from build123d import *

# Parameters (mm, degrees)
SKETCH_1_W             = 38
SKETCH_1_H             = 7
EXTRUDE_1_DEPTH        = 3
SKETCH_2_W             = 7
SKETCH_2_H             = 3
EXTRUDE_2_DEPTH        = 13
SKETCH_3_R             = 1.5
CUT_EXTRUDE_1_DEPTH    = 44.0464865
SKETCH_4_R             = 1.5
CUT_EXTRUDE_2_DEPTH    = 44.0464865
SKETCH_5_W             = 5
SKETCH_5_H             = 40.2
EXTRUDE_3_DEPTH        = 3
SKETCH_6_R             = 1.5
CUT_EXTRUDE_3_DEPTH    = 56.398916957
FILLET_1_R             = 5
FILLET_2_R             = 5
FILLET_2_OF_MIRROR_1_R = 5
SKETCH_7_W             = 73.096836427
SKETCH_7_H             = 5.118381576
CUT_EXTRUDE_4_DEPTH    = 13
SKETCH_9_W             = 54.2
SKETCH_9_H             = 3
EXTRUDE_4_DEPTH        = 1
SKETCH_8_R             = 1.5
CUT_EXTRUDE_5_DEPTH    = 61.669926652


with BuildPart() as part:
    # 草图1 → 凸台-拉伸1 (new body)
    with BuildSketch(Plane(origin=(0, 0, 0), x_dir=(1, 0, 0), z_dir=(0, 1, 0))):
        with Locations((-19, -3.5)):
            Rectangle(SKETCH_1_W, SKETCH_1_H)
    extrude_1 = extrude(amount=EXTRUDE_1_DEPTH)

    # 草图2 → 凸台-拉伸2 (add)
    with BuildSketch(Plane.XY.offset(7)):
        with Locations((-3.5, 1.5)):
            Rectangle(SKETCH_2_W, SKETCH_2_H)
    extrude(amount=EXTRUDE_2_DEPTH)

    # 草图3 → 切除-拉伸1 (cut, through all)
    with BuildSketch(Plane(origin=(0, 3, 0), x_dir=(1, 0, 0), z_dir=(0, 1, 0))):
        with Locations(Location((-3.5, -15, 0), (0, 0, 270))):
            Circle(SKETCH_3_R)
        with Locations(Location((-3.5, -5, 0), (0, 0, 270))):
            Circle(SKETCH_3_R)
    extrude(amount=-CUT_EXTRUDE_1_DEPTH, mode=Mode.SUBTRACT)

    # 草图4 → 切除-拉伸2 (cut, through all)
    with BuildSketch(Plane(origin=(0, 3, 0), x_dir=(1, 0, 0), z_dir=(0, 1, 0))):
        with Locations(Location((-33, -3.65, 0), (0, 0, 270))):
            Circle(SKETCH_4_R)
        with Locations(Location((-23, -3.65, 0), (0, 0, 270))):
            Circle(SKETCH_4_R)
    cut_extrude_2 = extrude(amount=-CUT_EXTRUDE_2_DEPTH, mode=Mode.SUBTRACT)

    # 草图5 → 凸台-拉伸3 (add)
    with BuildSketch(Plane(origin=(0, 3, 0), x_dir=(1, 0, 0), z_dir=(0, 1, 0))):
        with Locations((-15.5, 20.1)):
            Rectangle(SKETCH_5_W, SKETCH_5_H)
    extrude(amount=-EXTRUDE_3_DEPTH)

    # 草图6 → 切除-拉伸3 (cut, through all)
    with BuildSketch(Plane(origin=(0, 3, 0), x_dir=(1, 0, 0), z_dir=(0, 1, 0))):
        with Locations((-18, 1.5)):
            Circle(SKETCH_6_R)
    cut_extrude_3 = extrude(amount=-CUT_EXTRUDE_3_DEPTH, mode=Mode.SUBTRACT)

    # 圆角1
    fillet_1_edges = [part.edges().sort_by_distance(p)[0] for p in [
        (-7, 1.5, 7),
    ]]
    fillet(fillet_1_edges, radius=FILLET_1_R)

    # 圆角2
    fillet_2_edges = [part.edges().sort_by_distance(p)[0] for p in [
        (-13, 1.5, 0),
    ]]
    fillet(fillet_2_edges, radius=FILLET_2_R)

    # 镜向1: 凸台-拉伸1, 切除-拉伸2, 切除-拉伸3 across plane
    add(extrude_1.mirror(Plane(origin=(0, 0, -20.1), x_dir=(1, 0, 0), z_dir=(0, 0, -1))))
    add(cut_extrude_2.mirror(Plane(origin=(0, 0, -20.1), x_dir=(1, 0, 0), z_dir=(0, 0, -1))), mode=Mode.SUBTRACT)
    add(cut_extrude_3.mirror(Plane(origin=(0, 0, -20.1), x_dir=(1, 0, 0), z_dir=(0, 0, -1))), mode=Mode.SUBTRACT)

    # 圆角2 of 镜向1
    fillet_2_of_mirror_1_edges = [part.edges().sort_by_distance(p)[0] for p in [
        (-13, 1.5, -40.2),
    ]]
    fillet(fillet_2_of_mirror_1_edges, radius=FILLET_2_OF_MIRROR_1_R)

    # 草图7 → 切除-拉伸4 (cut)
    with BuildSketch(Plane(origin=(0, 0, 0), x_dir=(0, 0, -1), z_dir=(1, 0, 0))):
        with Locations((10.651581787, 2.559190788)):
            Rectangle(SKETCH_7_W, SKETCH_7_H)
    extrude(amount=-CUT_EXTRUDE_4_DEPTH, mode=Mode.SUBTRACT)

    # 草图9 → 凸台-拉伸4 (add)
    with BuildSketch(Plane(origin=(-13, 0, 0), x_dir=(0, 0, -1), z_dir=(1, 0, 0))):
        with Locations((20.1, 1.5)):
            Rectangle(SKETCH_9_W, SKETCH_9_H)
    extrude(amount=EXTRUDE_4_DEPTH)

    # 草图8 → 切除-拉伸5 (cut, through all)
    with BuildSketch(Plane(origin=(0, 3, 0), x_dir=(1, 0, 0), z_dir=(0, 1, 0))):
        with Locations(Location((-14.5, 14.1, 0), (0, 0, 270))):
            Circle(SKETCH_8_R)
        with Locations(Location((-14.5, 26.1, 0), (0, 0, 270))):
            Circle(SKETCH_8_R)
    extrude(amount=-CUT_EXTRUDE_5_DEPTH, mode=Mode.SUBTRACT)


solid = part.part
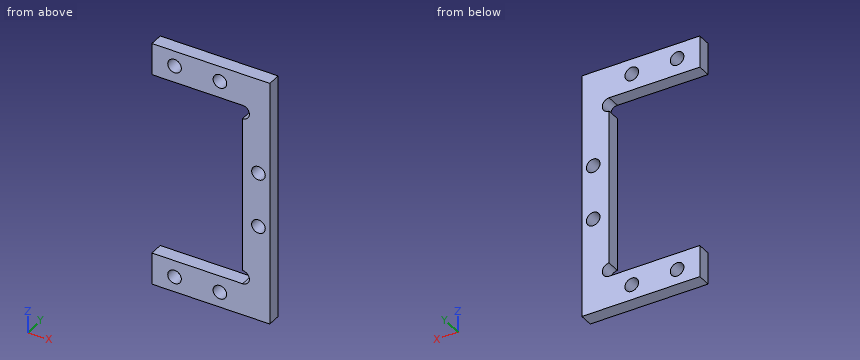
Here's how the part is built. I have some questions about the finished solid (model axes, mm). Round coordinates to 2 decimals unless told otherwise and drop trailing zeros. Loops run counter-clockwise (first coordinate to the right, second up) from the corner with the lowest first, then second, coordinate; pieces in that order, holes last. Notation, with made-up numbers: M 24,9.5 L 80,9.5 A8 ccw 80,23.5 Z; hole C -11,-26 d5. An arc over 180 degrees is marked long. Write each question's results on one line, items separated by ' | '. Start each with the question number.
(1) Will this pin go through, and if not, where does the flat tip stop? P1, Ø0.9, axis at y = 2, z = -15, coming from the -X side.
(2) If I drill on probe 1 along X at (y, z) = (2.3, -14); probe 2 along X at (y, z) = (1.7, -43.85); probe 3 along Z at (x, y) = (-26, 2.05), over which ranges is the centre line in solid material (lowest first)? Write a range as from..to.
(3) I want a section at A-A (x = -14.5). Please give me the cut outline in (y, z), then the cut area to 3 significant figures.
(4) I want a section at D-D (y = 1). Please give me the cut outline in (x, z).
(5) I want a section at B-B (x = -23). Please give me the cut outline in (y, z).
(6) I want a section at C-C (z = 3.65). Please give me the cut outline in (x, y), then the cut area to 3 significant figures.
Solved:
1) P1: stops at x = -18
2) probe 1: x = -18..-16, -13..-12 | probe 2: x = -38..-34.5, -31.5..-24.5, -21.5..-12 | probe 3: z = -47.2..-40.2, 0..7
3) outline: M 0,-47.2 L 3,-47.2 L 3,-27.6 L 0,-27.6 Z; M 0,-24.6 L 3,-24.6 L 3,-15.6 L 0,-15.6 Z; M 0,-12.6 L 3,-12.6 L 3,7 L 0,7 Z | area: 145 mm²
4) outline: M -38,-47.2 L -12,-47.2 L -12,7 L -38,7 L -38,0 L -18,0 A1.5 cw -18,-3 L -18,-37.2 A1.5 cw -18,-40.2 L -38,-40.2 Z; hole C -33,-43.85 d3; hole C -33,3.65 d3; hole C -23,-43.85 d3; hole C -23,3.65 d3; hole C -14.5,-26.1 d3; hole C -14.5,-14.1 d3
5) outline: M 0,-47.2 L 3,-47.2 L 3,-45.35 L 0,-45.35 Z; M 0,-42.35 L 3,-42.35 L 3,-40.2 L 0,-40.2 Z; M 0,0 L 3,0 L 3,2.15 L 0,2.15 Z; M 0,5.15 L 3,5.15 L 3,7 L 0,7 Z
6) outline: M -38,0 L -34.5,0 L -34.5,3 L -38,3 Z; M -31.5,0 L -24.5,0 L -24.5,3 L -31.5,3 Z; M -21.5,0 L -12,0 L -12,3 L -21.5,3 Z | area: 60.0 mm²
